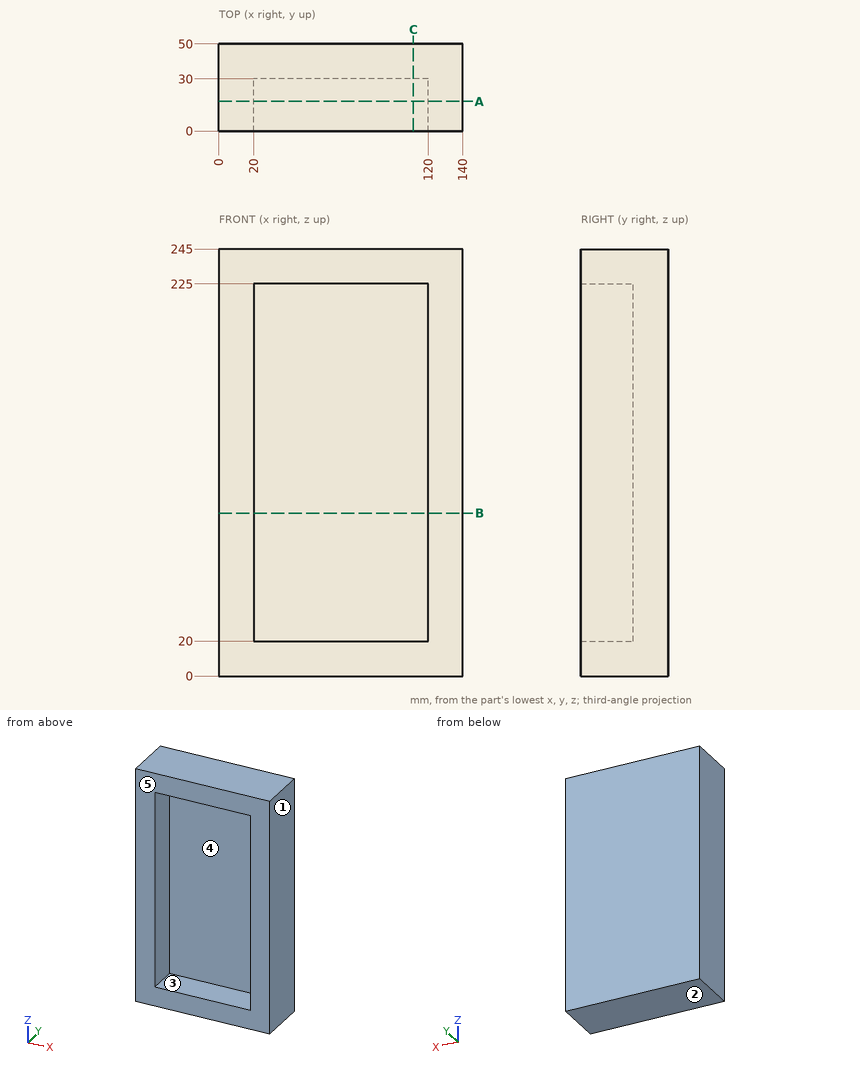
Input: dimensioned drawing with shaded views. Units: mm. Origin: part minimum x, y, z. A direction names the side the tool comes from. Give positions to 0.01 mm unless a question says otherwise; leave off trailing zeros. Order: outer loops, then holes, each group sorted by start corner. A loop starts at its lowest first (then second) coordinate and runs counter-clockwise, first axis right, second up.
(1) Contact query for a flat-ended pin moving along its axis: P1, Ø3, axis at x = 78.5, z = 98.5, coming from the -Y side. Output: stop coordinate, or through.
(2) Section query B-B (z = 93.5). Return the cut outline in (x, y).
(3) Section query A-A (y = 17). Return the cut outline in (x, z).
(4) Pull-direction query (X, two-part tool) for the marked faces 1, 2 and 3; classes: +X half, -X half, draft (parallel to the pull), parting line (faces both ways), or undercut.
(5) Access query for the marked faces 4 and 5. Directions: +Z, -Z, +X, -X, +Y, -Y. A direction counts if a zero-diameter tool reaches every point of the face in a straight line with its end or side. Return the directions, or none.
(6) Material intervals for line 1 along Z through (x, y) = (65, 10); line 2 along X through (y, z) = (26.5, 68.5); line 3 along Y through (x, z) = (105.5, 149), sorted ascending.
(7) Section query C-C (x = 111.5). Return the cut outline in (y, z).
Outcome:
1. P1: stops at y = 30
2. outline: (0, 0) - (20, 0) - (20, 30) - (120, 30) - (120, 0) - (140, 0) - (140, 50) - (0, 50) - close
3. outline: (0, 0) - (140, 0) - (140, 245) - (0, 245) - close; hole (20, 20) - (120, 20) - (120, 225) - (20, 225) - close
4. face 1: +X half
4. face 2: draft
4. face 3: undercut
5. face 4: -Y
5. face 5: +Z, -Z, +X, -X, -Y
6. line 1: z = 0 to 20, 225 to 245
6. line 2: x = 0 to 20, 120 to 140
6. line 3: y = 30 to 50
7. outline: (0, 0) - (50, 0) - (50, 245) - (0, 245) - (0, 225) - (30, 225) - (30, 20) - (0, 20) - close
